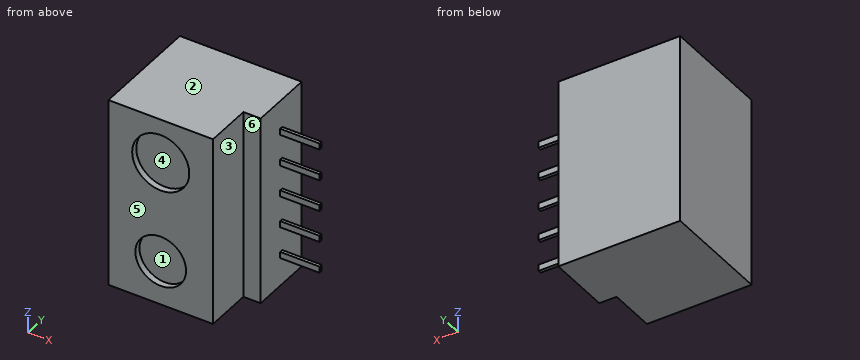
from build123d import *

# Parameters (mm, degrees)
SKETCH1_W           = 8.24
SKETCH1_H           = 15
BOSS_EXTRUDE1_DEPTH = 3.7
BOSS_EXTRUDE2_DEPTH = 5
SKETCH3_W           = 0.5
SKETCH3_H           = 0.25
BOSS_EXTRUDE3_DEPTH = 3.1
SKETCH4_R           = 2.25
SKETCH4_R_2         = 2
CUT_EXTRUDE1_DEPTH  = 0.5


with BuildPart() as part:
    # Sketch1 → Boss-Extrude1 (new body)
    with BuildSketch(Plane(origin=(0, 0, 0), x_dir=(1, 0, 0), z_dir=(0, 1, 0))):
        with Locations((-16.236881088, -0.721940399)):
            Rectangle(SKETCH1_W, SKETCH1_H)
    extrude(amount=BOSS_EXTRUDE1_DEPTH)

    # Sketch2 → Boss-Extrude2 (add)
    with BuildSketch(Plane(origin=(0, 3.7, 0), x_dir=(1, 0, 0), z_dir=(0, 1, 0))):
        Polygon((-20.356881088, -8.221940399), (-12.116881088, -8.221940399), (-10.756881088, -8.221940399), (-10.756881088, 6.778059601), (-12.116881088, 6.778059601), (-20.356881088, 6.778059601), align=None)
    extrude(amount=BOSS_EXTRUDE2_DEPTH)

    # Sketch3 → Boss-Extrude3 (add)
    with BuildSketch(Plane(origin=(-10.756881088, 0, 0), x_dir=(0, 0, -1), z_dir=(1, 0, 0))):
        with Locations((-5.721940399, 6.2)):
            Rectangle(SKETCH3_W, SKETCH3_H)
        with Locations((-3.221940399, 6.2)):
            Rectangle(SKETCH3_W, SKETCH3_H)
        with Locations((-0.721940399, 6.2)):
            Rectangle(SKETCH3_W, SKETCH3_H)
        with Locations((1.778059601, 6.2)):
            Rectangle(SKETCH3_W, SKETCH3_H)
        with Locations((4.278059601, 6.2)):
            Rectangle(SKETCH3_W, SKETCH3_H)
    extrude(amount=BOSS_EXTRUDE3_DEPTH)

    # Sketch4 → Cut-Extrude1 (cut)
    with BuildSketch(Plane(origin=(0, 0, 0), x_dir=(-1, 0, 0), z_dir=(0, -1, 0))):
        with Locations((16.236881088, -4.721940399)):
            Circle(SKETCH4_R)
        with Locations((16.236881088, 3.278059601)):
            Circle(SKETCH4_R_2)
    extrude(amount=-CUT_EXTRUDE1_DEPTH, mode=Mode.SUBTRACT)


solid = part.part
Geometry: final body of the model. Coordinates: model frame, mm. Face numbers are marked on the shaded views. A direction names the side the tool comes from. Give positions to 0.01 mm unless a question says otherwise; leave off trailing zeros. Loops run counter-clockwise (first coordinate to the right, second up) from the corner with the lowest first, then second, coordinate; pieces in that order, holes last. Notation, with made-up numbers: (80.25, -17.75) - (115.25, -17.75) arc R15 ccw to (115.25, 11.25) - close; hole circle Ø10 at (25.5, 38). An arc over 180 degrees is marked (long way). Answer as CSV lines item,"result". Start each with the question number.
1. Ray query, L1, parallel to X at y = 5.75, z = 7; L2, parallel to X at y = 1.25, z = -5.5; L3, parallel to Y at x = -14.5, z = 6. Return the intervals inside material, ascending.
2. Pin query (flat end, axial travel): P1, Ø2, axis at y = 2.5, z = 4.5, coming from the +X side; P2, Ø1.5, axis at x = -12, z = 6, coming from the -Y side; P3, Ø1.2, axis at x = -16.5, z = -4, coming from the -Y side; P4, Ø0.6, axis at x = -9, z = 1, coming from the +Y side (3 decimals). Return the tip coordinate at first contact, or that it passes through.
3. Section B-B, the plane z = 6.75. Return loops of the section in (x, y).
4. Reachability of the marked faces 5 and 6 from +Z, -Z, +X, -X, +Y, -Y: full face, straight path, thin tool, end or side. Return the list, or none.
5. Draft query along X for the marked faces 1, 2, 3 and 4. Return one class per face: released by +X, released by -X, zero draft, split by the parting line, or undercut.
6. Section D-D, the plane x = -11.5. Return loops of the section in (y, z).
7. Section A-A, the plane x = -9. Return loops of the section in (y, z) (3 decimals).
8. Section C-C, the plane y = 5. Return loops of the section in (x, z).
Answers:
1,L1,"x = -20.36 to -10.76"
1,L2,"x = -20.36 to -12.12"
1,L3,"y = 0.5 to 8.7"
2,P1,"stops at x = -12.12"
2,P2,"stops at y = 0"
2,P3,"stops at y = 0.5"
2,P4,"stops at y = 6.325"
3,outline,"(-20.36, 0) - (-17.21, 0) - (-17.21, 0.5) - (-15.26, 0.5) - (-15.26, 0) - (-12.12, 0) - (-12.12, 3.7) - (-10.76, 3.7) - (-10.76, 8.7) - (-20.36, 8.7) - close"
4,face 5,"+Z, -Z, +X, -X, -Y"
4,face 6,"+Z, -Z, +X, -Y"
5,face 1,"undercut"
5,face 2,"zero draft"
5,face 3,"released by +X"
5,face 4,"undercut"
6,outline,"(3.7, -6.78) - (8.7, -6.78) - (8.7, 8.22) - (3.7, 8.22) - close"
7,outline,"(6.075, -4.528) - (6.325, -4.528) - (6.325, -4.028) - (6.075, -4.028) - close; (6.075, -2.028) - (6.325, -2.028) - (6.325, -1.528) - (6.075, -1.528) - close; (6.075, 0.472) - (6.325, 0.472) - (6.325, 0.972) - (6.075, 0.972) - close; (6.075, 2.972) - (6.325, 2.972) - (6.325, 3.472) - (6.075, 3.472) - close; (6.075, 5.472) - (6.325, 5.472) - (6.325, 5.972) - (6.075, 5.972) - close"
8,outline,"(-20.36, -6.78) - (-10.76, -6.78) - (-10.76, 8.22) - (-20.36, 8.22) - close"
